Can you work these out from the model? Positions are in its coordinate system, mm. Face numbers are marked on the shaded views. Coordinates: 2 decimals unless noted, no trailing zeros. Write each loop counter-clockwise with the first axis right and the second up, starting at its lowest first coordinate (ties: lowest second). Pieces come first, ordered by that corner, then holes. Notation, with made-up numbers: (35.25, 42.5) - (77.25, 42.5) arc R14 cw to (77.25, 62.5) - close; hole circle Ø1 at (-6.5, 43.5). An arc over 180 degrees is marked (long way). Use one line per item in the form item = value. Start each with the question number.
(1) If we section it at B-B on z = 0: Please give me the cut outline in (x, y).
(2) Thinking about a two-plate mould opening in Z: for the marked faces 1, 2 and 3, which applies, pulls with the +Z half, pulls with the -Z half, needs draft (parallel to the pull), parting line crosses it, or undercut?
(3) If we section it at A-A on y = 57.5: Please give me the cut outline in (x, z), then the cut area to 3 significant figures.
(4) If we section it at D-D on z = -127.5: Please give me the cut outline in (x, y).
(5) If I drill on probe 1 along X at (y, z) = (1, 0); probe 2 along Z at (x, y) = (6.5, 63.5); probe 3 along Y at (x, z) = (-3, -111), over which ranges is the centre line in solid material (lowest first)? Write a range as from..to.
(6) If we section it at C-C on x = 0: Please give me the cut outline in (y, z).
(7) For pin 1 Ø4 at (x, y) = (-1, 26) entering from -Z; pin 2 Ø2 at (x, z) = (-2, -140.5) entering from -Y; pin 3 Ø5 at (x, z) = (-3, -55.5) entering from -Y, each with a flat end and sliding along its axis, tell me the tip position at first contact or that it passes through.
```python
from build123d import *

# Parameters (mm, degrees)
SKETCH1_W                    = 17.5
SKETCH1_H                    = 10
BASE_FLANGE1_DEPTH           = 2
EDGE_FLANGE1_DEPTH           = 17.5
EDGE_FLANGE2_STRIP_W         = 9.4732
EDGE_FLANGE2_STRIP_H         = 2
EDGE_FLANGE2_STRIP_CUT_DEPTH = 17.5
EDGE_FLANGE2_DEPTH           = 17.5
EDGE_FLANGE3_STRIP_W         = 9.4732
EDGE_FLANGE3_STRIP_H         = 2
EDGE_FLANGE3_STRIP_CUT_DEPTH = 17.5
EDGE_FLANGE3_DEPTH           = 17.5
SKETCH18_R                   = 4
CUT_EXTRUDE2_DEPTH           = 2
F_4_CLEARANCE_HOLE1_D        = 3.2639
F_4_CLEARANCE_HOLE1_DEPTH    = 2
F_4_CLEARANCE_HOLE1_TIP      = 0.980574487
CUT_EXTRUDE3_DEPTH           = 2


# Sheet-metal steps are written as plain solids
with BuildPart() as part:
    # Sketch1 → Base-Flange1 (new body)
    with BuildSketch(Plane(origin=(0, 0, 0), x_dir=(1, 0, 0), z_dir=(0, 1, 0))):
        Rectangle(SKETCH1_W, SKETCH1_H)
    extrude(amount=BASE_FLANGE1_DEPTH)

    # Edge-Flange1 section (across the edge) → Edge-Flange1 (add)
    with BuildSketch(Plane(origin=(-8.75, 2, 5.7366), x_dir=(0, 0, -1), z_dir=(1, 0, 0))):
        with BuildLine():
            Line((-2, 0.7366), (-2, 66))
            Line((-2, 66), (0, 66))
            Line((0, 66), (0, 0.7366))
            ThreePointArc((0, 0.7366), (0.215745145, 0.215745145), (0.7366, 0))
            Line((0.7366, 0), (0.7366, -2))
            ThreePointArc((0.7366, -2), (-1.198468417, -1.198468417), (-2, 0.7366))
        make_face()
    extrude(amount=EDGE_FLANGE1_DEPTH)

    # Edge-Flange2 strip (across the edge) → Edge-Flange2 strip cut (cut)
    with BuildSketch(Plane(origin=(-8.75, 68, 5.7366), x_dir=(0, -1, 0), z_dir=(1, 0, 0))):
        with Locations((-2, -1)):
            Rectangle(EDGE_FLANGE2_STRIP_W, EDGE_FLANGE2_STRIP_H)
    extrude(amount=EDGE_FLANGE2_STRIP_CUT_DEPTH, mode=Mode.SUBTRACT)

    # Edge-Flange2 section (across the edge) → Edge-Flange2 (add)
    with BuildSketch(Plane(origin=(-8.75, 68, 5.7366), x_dir=(0, -1, 0), z_dir=(1, 0, 0))):
        with BuildLine():
            Line((0, 0.7366), (0, 147))
            Line((0, 147), (2, 147))
            Line((2, 147), (2, 0.7366))
            ThreePointArc((2, 0.7366), (2.215745145, 0.215745145), (2.7366, 0))
            Line((2.7366, 0), (2.7366, -2))
            ThreePointArc((2.7366, -2), (0.801531583, -1.198468417), (0, 0.7366))
        make_face()
    extrude(amount=EDGE_FLANGE2_DEPTH)

    # Edge-Flange3 strip (across the edge) → Edge-Flange3 strip cut (cut)
    with BuildSketch(Plane(origin=(-8.75, 66, -141.2634), x_dir=(0, 0, 1), z_dir=(1, 0, 0))):
        with Locations((-2, -1)):
            Rectangle(EDGE_FLANGE3_STRIP_W, EDGE_FLANGE3_STRIP_H)
    extrude(amount=EDGE_FLANGE3_STRIP_CUT_DEPTH, mode=Mode.SUBTRACT)

    # Edge-Flange3 section (across the edge) → Edge-Flange3 (add)
    with BuildSketch(Plane(origin=(-8.75, 66, -141.2634), x_dir=(0, 0, 1), z_dir=(1, 0, 0))):
        with BuildLine():
            Line((0, 0.7366), (0, 16))
            Line((0, 16), (2, 16))
            Line((2, 16), (2, 0.7366))
            ThreePointArc((2, 0.7366), (2.215745145, 0.215745145), (2.7366, 0))
            Line((2.7366, 0), (2.7366, -2))
            ThreePointArc((2.7366, -2), (0.801531583, -1.198468417), (0, 0.7366))
        make_face()
    extrude(amount=EDGE_FLANGE3_DEPTH)

    # Sketch18 → Cut-Extrude2 (cut)
    with BuildSketch(Plane(origin=(0, 0, -141.2634), x_dir=(-1, 0, 0), z_dir=(0, 0, -1))):
        with Locations(Location((0, 57.5, 0), (0, 0, 90))):
            Circle(SKETCH18_R)
    extrude(amount=-CUT_EXTRUDE2_DEPTH, mode=Mode.SUBTRACT)

    # #4 Clearance Hole1
    with Locations(Plane.XZ):
        with Locations((4.75, 0), (-4.75, 0)):
            Hole(F_4_CLEARANCE_HOLE1_D / 2, depth=F_4_CLEARANCE_HOLE1_DEPTH)
            with Locations((0, 0, -(F_4_CLEARANCE_HOLE1_DEPTH + F_4_CLEARANCE_HOLE1_TIP / 2))):  # 118° drill point
                Cone(0, F_4_CLEARANCE_HOLE1_D / 2, F_4_CLEARANCE_HOLE1_TIP, mode=Mode.SUBTRACT)

    # Sketch23 → Cut-Extrude3 (cut)
    with BuildSketch(Plane.XZ.offset(-66)):
        with BuildLine():
            Line((-1.65, -61.0268), (-1.65, -56.0268))
            ThreePointArc((-1.65, -56.0268), (0, -54.3768), (1.65, -56.0268))
            Line((1.65, -56.0268), (1.65, -61.0268))
            ThreePointArc((1.65, -61.0268), (0, -62.6768), (-1.65, -61.0268))
        make_face()
    extrude(amount=-CUT_EXTRUDE3_DEPTH, mode=Mode.SUBTRACT)


solid = part.part
```
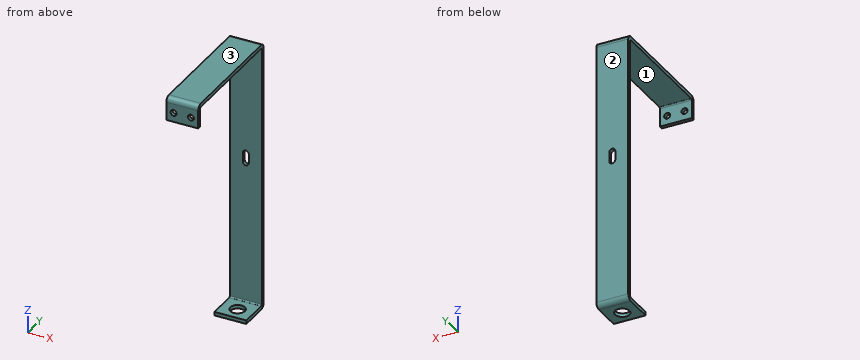
Reported:
q1.outline = (-8.75, 0) - (-6.38, 0) - (-6.38, 2) - (-8.75, 2) - close; (-8.75, 66) - (8.75, 66) - (8.75, 68) - (-8.75, 68) - close; (-3.12, 0) - (3.12, 0) - (3.12, 2) - (-3.12, 2) - close; (6.38, 0) - (8.75, 0) - (8.75, 2) - (6.38, 2) - close
q2.face_1 = undercut
q2.face_2 = needs draft
q2.face_3 = pulls with the +Z half
q3.outline = (-8.75, -141.26) - (-4, -141.26) - (-4, -139.26) - (-8.75, -139.26) - close; (-8.75, 5.74) - (8.75, 5.74) - (8.75, 7.74) - (-8.75, 7.74) - close; (4, -141.26) - (8.75, -141.26) - (8.75, -139.26) - (4, -139.26) - close
q3.area = 54.0 mm2
q4.outline = (-8.75, 66) - (8.75, 66) - (8.75, 68) - (-8.75, 68) - close
q5.probe_1 = -8.75..-6.38, -3.12..3.12, 6.38..8.75
q5.probe_2 = -141.26..-139.26, 5.74..7.74
q5.probe_3 = 66..68
q6.outline = (0, -5) - (2, -5) - (2, 5) arc R0.74 cw to (2.74, 5.74) - (65.26, 5.74) arc R0.74 cw to (66, 5) - (66, -54.38) - (68, -54.38) - (68, 5) arc R2.74 ccw to (65.26, 7.74) - (2.74, 7.74) arc R2.74 ccw to (0, 5) - close; (50, -141.26) - (53.5, -141.26) - (53.5, -139.26) - (50, -139.26) - close; (61.5, -141.26) - (65.26, -141.26) arc R2.74 ccw to (68, -138.53) - (68, -62.68) - (66, -62.68) - (66, -138.53) arc R0.74 cw to (65.26, -139.26) - (61.5, -139.26) - close
q7.pin_1 = 5.74
q7.pin_2 = 50
q7.pin_3 = 66
